Check sheet for the modelled part. Datum: model origin and axes. Units: mm. Give positions to 0.01 mm unless a question says otherwise; leave off trailing zeros. Write each loop counter-clockwise with the first axis right and the second up, starting at its lowest first coordinate (ties: lowest second). Pieces come first, ordered by that corner, then holes. Notation, with made-up numbers: (89.25, 75.25) -> (125.25, 75.25) arc R20 cw to (125.25, 82.25) -> close; hole circle Ø5 at (41, -11). An arc over 180 degrees is marked (long way). Use a Markdown table: item, result. Add a question column.
1. Cross-section at A-A (z = -23.5). Enter the section's corners in (x, y) (3 decimals), then the cut area to 3 significant figures.
2. Scan lines: probe 1 along Y at (x, z) = (194, -18.5); probe 2 along Y at (x, z) = (69, 5.5); probe 3 along Z at (x, y) = (151, 3.5). Record each from-to range of solid material in increasing order. Write a range as [from, to].
3. Cross-section at B-B (y = 30). Enter the section's corners in (x, z).
4. Cross-section at C-C (x = 195). Enter the section's corners in (y, z).
5. Gauge pin test, flat ends, axial feed: P1, Ø10, axis at x = 219.5, z = -47.5, coming from the -Y side; P2, Ø12, axis at x = 106, y = 17.5, coming from the +Z side; P3, Ø5, axis at x = 214, z = -40.5, coming from the +Y side; P4, Ø1.5, axis at x = 48.5, z = 8.5, coming from the +Y side. Record the tip position at first contact, or that the pin passes through.
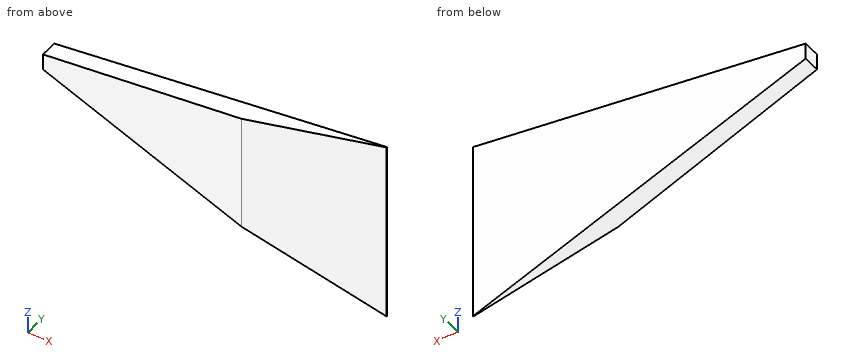
Autodesk Inventor part; units mm, degrees
ref_plane "CP1_XY" through (0, 0, 0) normal (0, 0, 1) x (1, 0, 0)
ref_plane "CP1_YZ" through (0, 0, 0) normal (1, 0, 0) x (0, 1, 0)
ref_plane "CP1_ZX" through (0, 0, 0) normal (0, 1, 0) x (0, 0, 1)
sketch "Sketch_4" plane through (0, 0, 0) normal (0, 0, 1) x (1, 0, 0)
  line L0 (-1.9813, 35.0728) -> (-1.9773, 23.1005)
  line L1 (-1.9773, 23.1005) -> (150, 0)
  line L2 (150, 0) -> (250, 0)
  line L3 (250, 0) -> (250, 0.375)
  line L4 (250, 0.375) -> (-1.9813, 35.0728)
extrude "Extrusion1" add sketch "Sketch_4" along normal mid plane 129
sketch "Sketch_5" plane through (0, 0, 0) normal (0, 1, 0) x (-1, 0, 0)
  line L0 (5, 131) -> (-260, 131)
  line L1 (-260, 131) -> (-260, -131)
  line L2 (-260, -131) -> (5, -131)
  line L3 (5, -131) -> (5, 131)
  line L4 (2.9262, 5.3387) -> (-250, 62.5)
  line L5 (-250, 62.5) -> (-250, -62.5)
  line L6 (-250, -62.5) -> (2.9262, -5.3387)
  line L7 (2.9262, -5.3387) -> (2.9262, 5.3387)
extrude "Extrusion2" cut sketch "Sketch_5" along normal mid plane 91.6
ref_plane "CP1_XY" through (0, 0, 0) normal (0, 0, 1) x (1, 0, 0)
ref_plane "CP1_YZ" through (0, 0, 0) normal (1, 0, 0) x (0, 1, 0)
ref_plane "CP1_ZX" through (0, 0, 0) normal (0, 1, 0) x (0, 0, 1)
properties part number "Receivingbeam_OXS200_11728845"
Worked answers:
| question | item | result |
|---|---|---|
| 1 | outline | (77.434, 11.03) -> (150, 0) -> (250, 0) -> (250, 0.375) -> (77.434, 24.137) -> close |
| 1 | area | 1,710 mm² |
| 2 | probe 1 | y = [0, 8.09] |
| 2 | probe 2 | y = [12.31, 25.3] |
| 2 | probe 3 | z = [-40.13, 40.13] |
| 3 | outline | (-1.98, -5.55) -> (34.86, -13.88) -> (34.86, 13.88) -> (-1.98, 5.55) -> close |
| 4 | outline | (0, -50.07) -> (7.95, -50.07) -> (7.95, 50.07) -> (0, 50.07) -> close |
| 5 | P1 | stops at y = 0 |
| 5 | P2 | stops at z = 31.31 |
| 5 | P3 | stops at y = 5.68 |
| 5 | P4 | stops at y = 28.22 |
